Job drawing, mm, ordinate dimensions from the low corner. One solid piece. A direction names the side the tool comes from. Round coordinates to 2 decimals unless told otherwise and drop trailing zeros. Loops run counter-clockwise (first coordinate to the right, second up) from the corner with the lowest first, then second, coordinate; pieces in that order, holes last. Notation, with made-up numbers: M -35,68 L -28,68 A5 cw -28,77 Z; hole C -36.75,14 d6. An arc over 180 degrees is marked long. One line per item, written item: value.
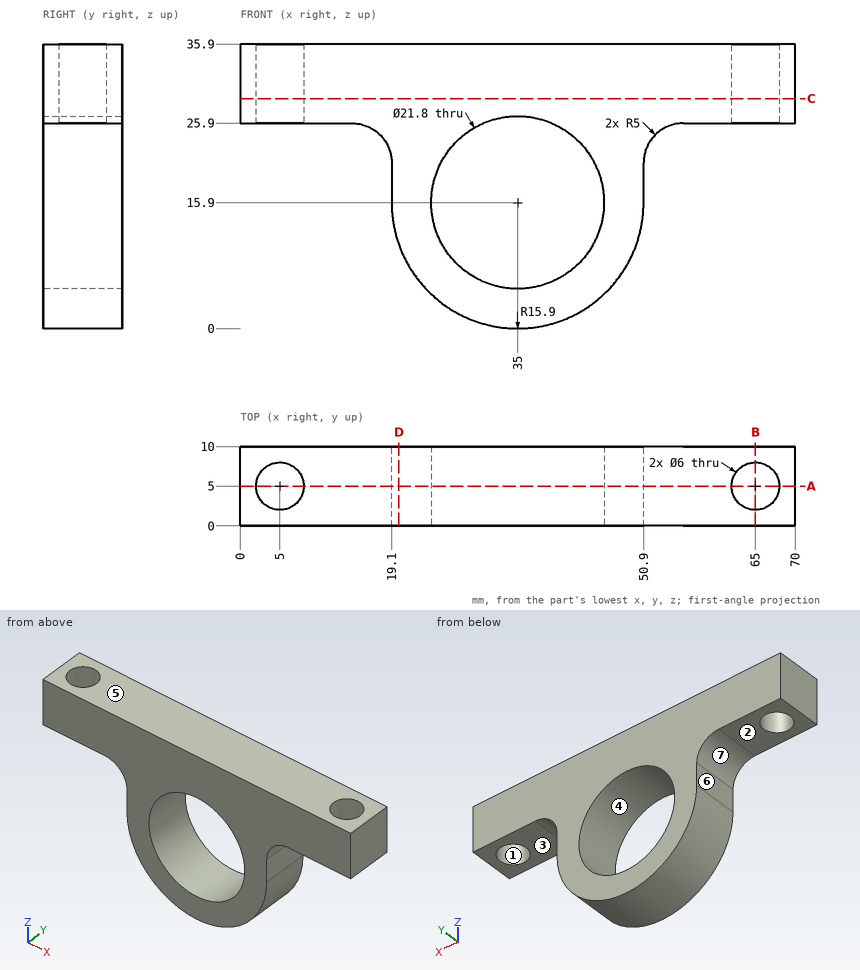
Item 1: Slice it at B-B, the plane x = 65. Give the cut face in (y, z).
Check values:
outline: M 0,25.9 L 2,25.9 L 2,35.9 L 0,35.9 Z; M 8,25.9 L 10,25.9 L 10,35.9 L 8,35.9 Z
Item 2: Wall check: line 1 along Y through (x, z) = (5, 30); line 2 along X through (y, z) = (5.75, 15.9); line 3 along X through (y, z) = (7.5, 30). Give the ranges that are in metal, low to high.
Check values:
line 1: y = 0 to 2, 8 to 10
line 2: x = 19.1 to 24.1, 45.9 to 50.9
line 3: x = 0 to 3.34, 6.66 to 63.34, 66.66 to 70
Item 3: Slice it at A-A, the plane y = 5. Give the cut face in (x, z).
Check values:
outline: M 0,25.9 L 2,25.9 L 2,35.9 L 0,35.9 Z; M 8,25.9 L 14.1,25.9 A5 cw 19.1,20.9 L 19.1,15.9 A15.9 ccw 50.9,15.9 L 50.9,20.9 A5 cw 55.9,25.9 L 62,25.9 L 62,35.9 L 8,35.9 Z; M 68,25.9 L 70,25.9 L 70,35.9 L 68,35.9 Z; hole C 35,15.9 d21.8
Item 4: Pull direction Z, two halves, no side cores. Call the marked faces 4, 5, 6 and 7: pulls with the +Z half, pulls with the -Z half, needs draft (parallel to the pull), parting line crosses it, or undercut.
Check values:
face 4: undercut
face 5: pulls with the +Z half
face 6: needs draft
face 7: pulls with the -Z half
Item 5: Which spindle directions (+Z, -Z, +X, -X, +Y, -Y) get a long thin tool onto all of the face, cutting with end or side? Do the marked faces 1, 2 and 3. Say none if no direction does.
Check values:
face 1: +Z, -Z
face 2: -Z, -X, +Y, -Y
face 3: -Z, +X, +Y, -Y
Item 6: Drop flat-ended pins along their axis: P1, Ø2.5, axis at y = 4, z = 19, coming from the -X side; P2, Ø5.5, axis at y = 6, z = 18, coming from the +X side; P3, Ø13, axis at x = 35, z = 15.9, coming from the +Y side; P4, Ø5, axis at x = 8, y = 4.5, coming from the -Z side. Give the stop position or say it passes through.
Check values:
P1: stops at x = 19.1
P2: stops at x = 50.9
P3: passes through
P4: stops at z = 25.9
Item 7: Slice it at D-D, the plane x = 20. Give the cut face in (y, z), and give its area (3 significant figures).
Check values:
outline: M 0,10.63 L 10,10.63 L 10,35.9 L 0,35.9 Z
area: 253 mm2
Item 8: Slice it at C-C, the plane z = 29. Give the cut face in (x, y).
Check values:
outline: M 0,0 L 70,0 L 70,10 L 0,10 Z; hole C 5,5 d6; hole C 65,5 d6
